Verification items for this drawing (mm, ordinates from the low corner). Coordinates: 2 decimals unless noted, no trailing zeros. Order: outer loops, then holes, each group sorted by start corner. A loop starts at its lowest first (then second) coordinate and runs counter-clockwise, first axis right, second up.
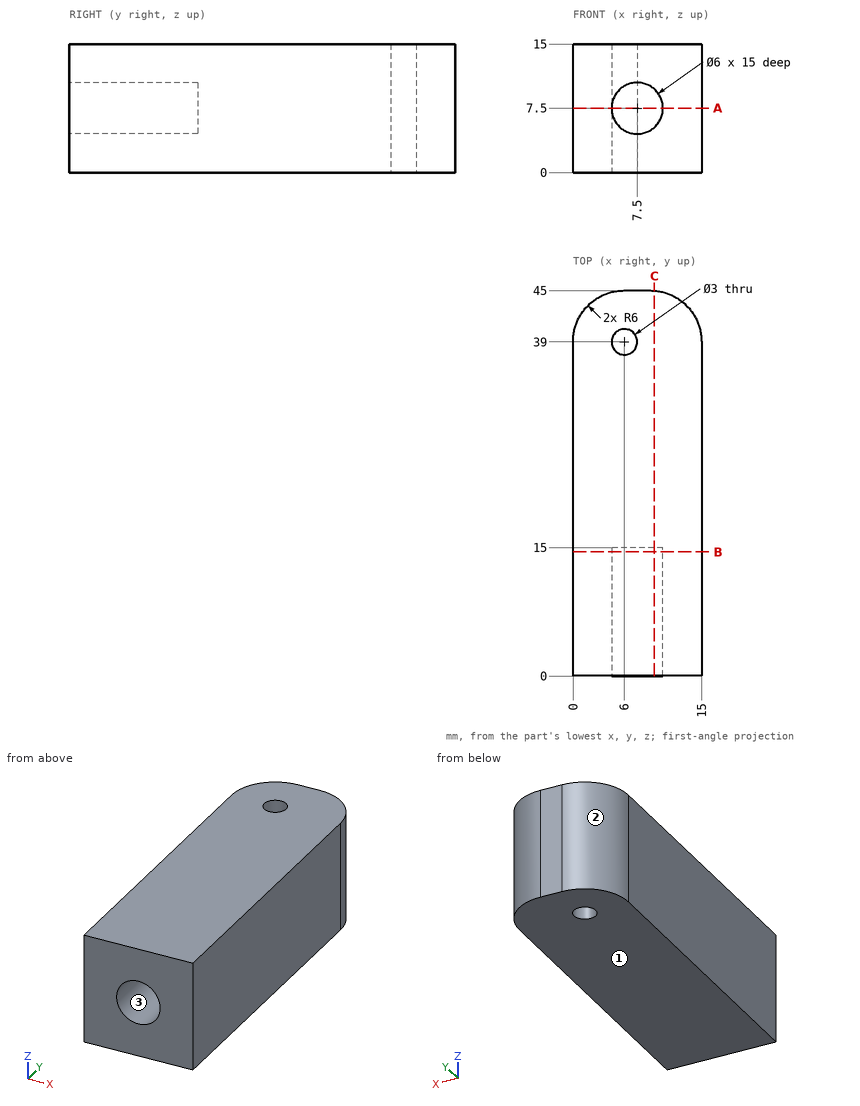
(1) Cross-section at A-A (z = 7.5). Enter the section's corners in (x, y).
Filled in:
outline: (0, 0) - (4.5, 0) - (4.5, 15) - (10.5, 15) - (10.5, 0) - (15, 0) - (15, 39) arc R6 ccw to (9, 45) - (6, 45) arc R6 ccw to (0, 39) - close; hole circle Ø3 at (6, 39)
(2) Release check for a two-part mould opening along X. For the marked faces 1, 2 and 3 record: +X half, -X half, draft (parallel to the pull), parting line (faces both ways), or undercut.
Filled in:
face 1: draft
face 2: -X half
face 3: undercut
(3) Cross-section at B-B (y = 14.5). Enter the section's corners in (x, z).
Filled in:
outline: (0, 0) - (15, 0) - (15, 15) - (0, 15) - close; hole circle Ø6 at (7.5, 7.5)
(4) Cross-section at C-C (x = 9.5). Enter the section's corners in (y, z), and give its area (3 significant figures).
Filled in:
outline: (0, 0) - (44.98, 0) - (44.98, 15) - (0, 15) - (0, 9.74) - (15, 9.74) - (15, 5.26) - (0, 5.26) - close
area: 608 mm2
(5) Go/stop test with a flat-tipped pin: P1, Ø5.5, axis at x = 7.5, z = 7.5, coming from the -Y side. Record where the tip stops, or that it passes through.
Filled in:
P1: stops at y = 15
(6) Thickness scan on probe 1 along Z at (x, y) = (7.5, 8.5); probe 2 along Y at (x, z) = (6, 8); probe 3 along X at (y, z) = (4, 9.75). Record the ranges inside material, lowest first.
Filled in:
probe 1: z = 0 to 4.5, 10.5 to 15
probe 2: y = 15 to 37.5, 40.5 to 45
probe 3: x = 0 to 5.52, 9.48 to 15
